Geometry: final body of the model. Coordinates: model frame, mm. A direction names the side the tool comes from. Give positions to 0.01 mm unless a question says otherwise; leave off trailing zeros. Loops run counter-clockwise (first coordinate to the right, second up) from the corner with the lowest first, then second, coordinate; pieces in that order, holes last. Notation, with made-up numbers: M -25,25.5 L -11,25.5 A23 cw -11,58.5 Z; hole C 7,83 d7. An arc over 180 degrees is marked long. Put each result on its own line as item: value.
```python
from build123d import *

# Parameters (mm, degrees)
EXTRUDE_1_DEPTH     = 20
SKETCH_2_R          = 16.745148551
CUT_EXTRUDE_1_DEPTH = 133.554049902
M5X0_82_D           = 4.2
M5X0_82_DEPTH       = 9.5
M5X0_82_TIP         = 1.2618073
M5X0_81_D           = 4.2
M5X0_81_DEPTH       = 9.5
M5X0_81_TIP         = 1.2618073


with BuildPart() as part:
    # Эскиз1 → Бобышка-Вытянуть1 (new body)
    with BuildSketch(Plane.XY):
        with BuildLine():
            Line((0, 0), (128, 0))
            ThreePointArc((128, 0), (64, -28.045964869), (0, 0))
        make_face()
    extrude(amount=EXTRUDE_1_DEPTH)

    # Эскиз2 → Вырез-Вытянуть1 (cut, through all)
    with BuildSketch(Plane(origin=(0, 0, 0), x_dir=(0, 0, -1), z_dir=(1, 0, 0))):
        with Locations((-10, 14.6)):
            Circle(SKETCH_2_R)
    extrude(amount=CUT_EXTRUDE_1_DEPTH, mode=Mode.SUBTRACT)

    # Отверстие обработанное метчиком M5x0.82
    with Locations(Plane.XY.offset(20)):
        with Locations((39, -10)):
            Hole(M5X0_82_D / 2, depth=M5X0_82_DEPTH)
            with Locations((0, 0, -(M5X0_82_DEPTH + M5X0_82_TIP / 2))):  # 118° drill point
                Cone(0, M5X0_82_D / 2, M5X0_82_TIP, mode=Mode.SUBTRACT)

    # Отверстие обработанное метчиком M5x0.81
    with Locations(Plane.XY.offset(20)):
        with Locations((89, -10)):
            Hole(M5X0_81_D / 2, depth=M5X0_81_DEPTH)
            with Locations((0, 0, -(M5X0_81_DEPTH + M5X0_81_TIP / 2))):  # 118° drill point
                Cone(0, M5X0_81_D / 2, M5X0_81_TIP, mode=Mode.SUBTRACT)


solid = part.part
```
Item 1: Line query: probe 1 along X at (y, z) = (-10, 14); probe 2 along Y at (x, z) = (39, 16.75); probe 3 along X at (y, z) = (-10.25, 11). Output: solid intervals per line, ascending. Write a range as [from, to].
Output values:
probe 1: [10.93, 36.9], [41.1, 86.9], [91.1, 117.07]
probe 2: [-24.38, -12.1], [-7.9, -0.72]
probe 3: [11.26, 36.91], [41.09, 86.91], [91.09, 116.74]
Item 2: Mould query, pull axis Z, two halves, no side actions, for faces 3 (the conical face through (39.35, -9.89, 9.46)), 4 (the cylindrical face through (63.104, -2.145, 10.12)), 5 (the flat face through (65, -11, 0)). Classes: pulls with the +Z half, pulls with the -Z half, needs draft (parallel to the pull), parting line crosses it, or undercut.
Output values:
face 3: pulls with the +Z half
face 4: undercut
face 5: pulls with the -Z half
Item 3: Set-up query: faces 1 (the cylindrical face through (65.01, -28.04, 9.86)), 2 (the cylindrical face through (91.1, -9.91, 15.18)). Return all of +Z, -Z, +X, -X, +Y, -Y with unobstructed straight access to the full face (end or side cutting, diameter ignored); none if empty.
Output values:
face 1: +Z, -Z, -Y
face 2: +Z
Item 4: Section D-D on x = 113. Output: boundary loops of the cut face in (y, z), then the cut area to 3 significant figures.
Output values:
outline: M -12.94,0 L 0,0 L 0,1.8 A16.75 cw 0,18.2 L 0,20 L -12.94,20 Z
area: 235 mm²
Item 5: Section C-C on y = -20. Output: boundary loops of the cut face in (x, z).
Output values:
outline: M 27.45,0 L 100.55,0 L 100.55,20 L 27.45,20 Z
Item 6: Section B-B on z = 17. Output: boundary loops of the cut face in (x, y), then the cut area to 3 significant figures.
Output values:
outline: M 0.57,-0.61 A87.05 ccw 127.43,-0.61 Z; hole C 39,-10 d4.2; hole C 89,-10 d4.2
area: 2,380 mm²
Item 7: Section A-A on x = 69. Output: boundary loops of the cut face in (y, z), then the cut area to 3 significant figures.
Output values:
outline: M -27.9,0 L 0,0 L 0,1.8 A16.75 cw 0,18.2 L 0,20 L -27.9,20 Z
area: 534 mm²
Item 8: Pin query (flat end, axial travel): pin 1 Ø6 at (x, z) = (102, 10) entering from -Y; pin 2 Ø6 at (y, z) = (-3.5, 4) entering from +X; pin 3 Ø5 at (y, z) = (-19, 8) entering from -X. Return the tip coordinate at first contact, or that it passes through.
Output values:
pin 1: y = -20.7
pin 2: x = 127.4
pin 3: x = 20.68
